Build history of the part. All positions in model axes, mm. Face numbers are marked on the shaded views. A direction names the side the tool comes from. Coordinates: 2 decimals unless noted, no trailing zeros. Order: outer loops, then holes, each group sorted by start corner. A loop starts at its lowest first (then second) coordinate and runs counter-clockwise, first axis right, second up. Notation, with made-up numbers: (38, 57.5) - (58, 57.5) arc R14 cw to (58, 64.5) - close; hole circle Ø2 at (56.5, -14.75). An arc over 180 degrees is marked (long way). Return JSON: item names as keys, results as strings.
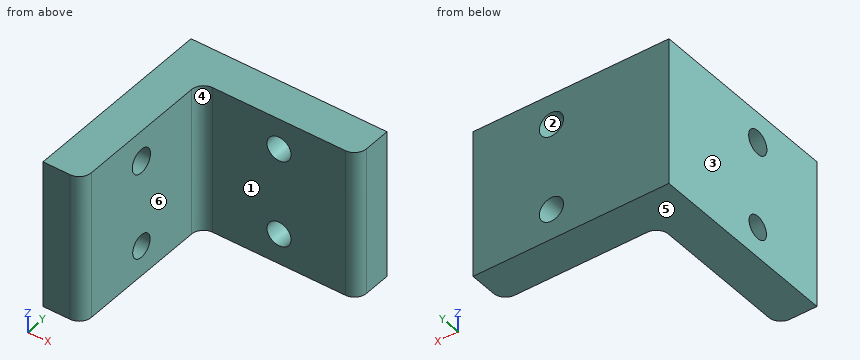
from build123d import *

# Parameters (mm, degrees)
SKETCH1_W           = 34.0614
SKETCH1_H           = 45
BOSS_EXTRUDE1_DEPTH = 8.9916
SKETCH2_W           = 34.0614
SKETCH2_H           = 8.9916
BOSS_EXTRUDE2_DEPTH = 36.0084
CUT_EXTRUDE2_REACH  = 10.992
SKETCH5_R           = 2.7686
SKETCH5_R_2         = 2.6416
CUT_EXTRUDE3_REACH  = 47
SKETCH6_R           = 2.7686
FILLET1_R           = 2.7686


with BuildPart() as part:
    # Sketch1 → Boss-Extrude1 (new body)
    with BuildSketch(Plane(origin=(0, 0, 0), x_dir=(0, 0, -1), z_dir=(1, 0, 0))):
        Rectangle(SKETCH1_W, SKETCH1_H)
    extrude(amount=BOSS_EXTRUDE1_DEPTH)

    # Sketch2 → Boss-Extrude2 (add)
    with BuildSketch(Plane(origin=(8.9916, 0, 0), x_dir=(0, 0, -1), z_dir=(1, 0, 0))):
        with Locations((0, 18.0042)):
            Rectangle(SKETCH2_W, SKETCH2_H)
    extrude(amount=BOSS_EXTRUDE2_DEPTH)

    # Sketch5 → Cut-Extrude2 (cut, up to next)
    with BuildSketch(Plane(origin=(8.9916, 0, 0), x_dir=(0, 0, -1), z_dir=(1, 0, 0)), mode=Mode.PRIVATE) as cut_extrude2_sk1:
        with Locations((-10.0076, -4.4958)):
            Circle(SKETCH5_R)
    cut_extrude2_tool1 = extrude(cut_extrude2_sk1.sketch, amount=-CUT_EXTRUDE2_REACH, mode=Mode.PRIVATE) & part.part
    add(cut_extrude2_tool1.solids().sort_by_distance((8.9916, -4.4958, 10.0076))[0], mode=Mode.SUBTRACT)
    # Sketch5 → Cut-Extrude2 (cut, up to next)
    with BuildSketch(Plane(origin=(8.9916, 0, 0), x_dir=(0, 0, -1), z_dir=(1, 0, 0)), mode=Mode.PRIVATE) as cut_extrude2_sk2:
        with Locations((10.0076, -4.4958)):
            Circle(SKETCH5_R_2)
    cut_extrude2_tool2 = extrude(cut_extrude2_sk2.sketch, amount=-CUT_EXTRUDE2_REACH, mode=Mode.PRIVATE) & part.part
    add(cut_extrude2_tool2.solids().sort_by_distance((8.9916, -4.4958, -10.0076))[0], mode=Mode.SUBTRACT)

    # Sketch6 → Cut-Extrude3 (cut, up to next)
    with BuildSketch(Plane(origin=(0, 22.5, 0), x_dir=(1, 0, 0), z_dir=(0, 1, 0)), mode=Mode.PRIVATE) as cut_extrude3_sk1:
        with Locations((26.995718, 10.0076)):
            Circle(SKETCH6_R)
    cut_extrude3_tool1 = extrude(cut_extrude3_sk1.sketch, amount=-CUT_EXTRUDE3_REACH, mode=Mode.PRIVATE) & part.part
    add(cut_extrude3_tool1.solids().sort_by_distance((26.995718, 22.5, -10.0076))[0], mode=Mode.SUBTRACT)
    # Sketch6 → Cut-Extrude3 (cut, up to next)
    with BuildSketch(Plane(origin=(0, 22.5, 0), x_dir=(1, 0, 0), z_dir=(0, 1, 0)), mode=Mode.PRIVATE) as cut_extrude3_sk2:
        with Locations((26.995718, -10.0076)):
            Circle(SKETCH6_R)
    cut_extrude3_tool2 = extrude(cut_extrude3_sk2.sketch, amount=-CUT_EXTRUDE3_REACH, mode=Mode.PRIVATE) & part.part
    add(cut_extrude3_tool2.solids().sort_by_distance((26.995718, 22.5, 10.0076))[0], mode=Mode.SUBTRACT)

    # Fillet1
    fillet1_edges = [part.edges().sort_by_distance(p)[0] for p in [
        (8.9916, -22.5, 0),
        (8.9916, 13.5084, 0),
        (45, 13.5084, 0),
    ]]
    fillet(fillet1_edges, radius=FILLET1_R)


solid = part.part
1. Tool access for the marked faces 5 and 6: list every direction of +Z, -Z, +X, -X, +Y, -Y with a clear straight run to the whole face (end or side of a thin tool).
Check values:
{"face 5": "-Z, +X, -X, +Y, -Y", "face 6": "+Z, -Z, +X, -Y"}
2. Cut at D-D on z = -0.5. Give the cut face in (x, y).
Check values:
{"outline": "(0, -22.5) - (6.22, -22.5) arc R2.77 ccw to (8.99, -19.73) - (8.99, 10.74) arc R2.77 cw to (11.76, 13.51) - (42.23, 13.51) arc R2.77 ccw to (45, 16.28) - (45, 22.5) - (0, 22.5) - close"}
3. Cut at A-A on z = 11. Give the cut face in (x, y), plus the area to 3 significant figures.
Check values:
{"outline": "(0, -22.5) - (6.22, -22.5) arc R2.77 ccw to (8.99, -19.73) - (8.99, -7.08) - (0, -7.08) - close; (0, -1.91) - (8.99, -1.91) - (8.99, 10.74) arc R2.77 cw to (11.76, 13.51) - (24.41, 13.51) - (24.41, 22.5) - (0, 22.5) - close; (29.58, 13.51) - (42.23, 13.51) arc R2.77 ccw to (45, 16.28) - (45, 22.5) - (29.58, 22.5) - close", "area": "634 mm²"}
4. Mould opens along X. For the marked faces 1, 2, 3 and 4 say: pulls with the +X half, pulls with the -X half, needs draft (parallel to the pull), parting line crosses it, or undercut.
Check values:
{"face 1": "needs draft", "face 2": "undercut", "face 3": "pulls with the -X half", "face 4": "pulls with the +X half"}
5. Cut at C-C on x = 26.5. Give the cut face in (y, z), plus the area to 3 significant figures.
Check values:
{"outline": "(13.51, -17.03) - (22.5, -17.03) - (22.5, -12.73) - (13.51, -12.73) - close; (13.51, -7.28) - (22.5, -7.28) - (22.5, 7.28) - (13.51, 7.28) - close; (13.51, 12.73) - (22.5, 12.73) - (22.5, 17.03) - (13.51, 17.03) - close", "area": "208 mm²"}
6. Cut at B-B on y = -5.5. Give the cut face in (x, z), plus the area to 3 significant figures.
Check values:
{"outline": "(0, -17.03) - (8.99, -17.03) - (8.99, -12.45) - (0, -12.45) - close; (0, -7.56) - (8.99, -7.56) - (8.99, 7.43) - (0, 7.43) - close; (0, 12.59) - (8.99, 12.59) - (8.99, 17.03) - (0, 17.03) - close", "area": "216 mm²"}
7. Drop flat-ended pins along their axis: pin 1 (9 mm diameter, centred on x = 27.5, z = 5, fed in from -Y); pin 2 (1 mm diameter, centred on y = -11, z = -2, fed in from +X). Give the stop position or say it passes through.
Check values:
{"pin 1": "y = 13.51", "pin 2": "x = 8.99"}
8. Probe L1, parallel to Y at x = 13.5, z = -3; L2, parallel to X at y = -18, z = 0; L3, parallel to X at y = 14.5, z = -2. List the from-to ranges inside material, lowest first.
Check values:
{"L1": "13.51 to 22.5", "L2": "0 to 8.99", "L3": "0 to 44.35"}
